```python
from build123d import *

# Parameters (mm, degrees)
SKETCH1_W                    = 68
SKETCH1_H                    = 40
BOSS_EXTRUDE1_DEPTH          = 3
SKETCH3_W                    = 50
SKETCH3_H                    = 42
BOSS_EXTRUDE2_DEPTH          = 3
CUT_EXTRUDE1_REACH           = 71.145
SKETCH4_R                    = 11.1
CSK_FOR_M3_SFHCS1_AT_2_COUNT = 2
CSK_FOR_M3_SFHCS1_AT_2_PITCH = 31
CSK_FOR_M3_SFHCS1_AT_3_COUNT = 2
CSK_FOR_M3_SFHCS1_AT_3_PITCH = 31
CSK_FOR_M3_SFHCS1_AT_4_COUNT = 2
CSK_FOR_M3_SFHCS1_AT_4_PITCH = 43.840620434
BOSS_EXTRUDE3_DEPTH          = 50
SKETCH9_W                    = 42.2
SKETCH9_H                    = 42
CUT_EXTRUDE2_DEPTH           = 37
FILLET1_R                    = 3
CSK_FOR_M3_SFHCS2_AT_2_COUNT = 2
CSK_FOR_M3_SFHCS2_AT_2_PITCH = 61.351446601
CSK_FOR_M3_SFHCS2_AT_3_COUNT = 2
CSK_FOR_M3_SFHCS2_AT_3_PITCH = 20
CSK_FOR_M3_SFHCS2_AT_4_COUNT = 2
CSK_FOR_M3_SFHCS2_AT_4_PITCH = 58


with BuildPart() as part:
    # Sketch1 → Boss-Extrude1 (new body)
    with BuildSketch(Plane.XY):
        with Locations((0, -20)):
            Rectangle(SKETCH1_W, SKETCH1_H)
    extrude(amount=BOSS_EXTRUDE1_DEPTH)

    # Sketch3 → Boss-Extrude2 (add)
    with BuildSketch(Plane(origin=(0, 0, 0), x_dir=(1, 0, 0), z_dir=(0, 1, 0))):
        with Locations((0, -24)):
            Rectangle(SKETCH3_W, SKETCH3_H)
    extrude(amount=-BOSS_EXTRUDE2_DEPTH)

    # Sketch4 → Cut-Extrude1 (cut, up to next)
    with BuildSketch(Plane(origin=(0, 0, 0), x_dir=(1, 0, 0), z_dir=(0, 1, 0)), mode=Mode.PRIVATE) as cut_extrude1_sk1:
        with Locations(Location((0, -24, 0), (0, 0, 180))):
            Circle(SKETCH4_R)
    cut_extrude1_tool1 = extrude(cut_extrude1_sk1.sketch, amount=-CUT_EXTRUDE1_REACH, mode=Mode.PRIVATE) & part.part
    add(cut_extrude1_tool1.solids().sort_by_distance((0, 0, 24))[0], mode=Mode.SUBTRACT)

    # Sketch6 → CSK for M3 SFHCS1 (revolve, cut)
    with BuildSketch(Plane(origin=(-15.5, 0, 8.5), x_dir=(0, 0, 1), z_dir=(1, 0, 0))):
        Polygon((0, 0), (0, 3), (1.7, 3), (1.7, 1.66), (3.36, 0), align=None)
    csk_for_m3_sfhcs1 = revolve(axis=Axis((-15.5, 6.35, 8.5), (0, -1, 0)), mode=Mode.SUBTRACT)

    # CSK for M3 SFHCS1 at 2: CSK for M3 SFHCS1 ×2
    with Locations(*[(i * CSK_FOR_M3_SFHCS1_AT_2_PITCH, 0, 0) for i in range(1, CSK_FOR_M3_SFHCS1_AT_2_COUNT)]):
        add(csk_for_m3_sfhcs1, mode=Mode.SUBTRACT)

    # CSK for M3 SFHCS1 at 3: CSK for M3 SFHCS1 ×2
    with Locations(*[(0, 0, i * CSK_FOR_M3_SFHCS1_AT_3_PITCH) for i in range(1, CSK_FOR_M3_SFHCS1_AT_3_COUNT)]):
        add(csk_for_m3_sfhcs1, mode=Mode.SUBTRACT)

    # CSK for M3 SFHCS1 at 4: CSK for M3 SFHCS1 ×2
    with Locations(*[Vector(0.7071067811865476, 0, 0.7071067811865476) * (i * CSK_FOR_M3_SFHCS1_AT_4_PITCH) for i in range(1, CSK_FOR_M3_SFHCS1_AT_4_COUNT)]):
        add(csk_for_m3_sfhcs1, mode=Mode.SUBTRACT)

    # Sketch7 → Boss-Extrude3 (add)
    with BuildSketch(Plane.ZY.offset(25)):
        Polygon((45, -3), (3, -36.75), (3, -3), align=None)
    extrude(amount=-BOSS_EXTRUDE3_DEPTH)

    # Sketch9 → Cut-Extrude2 (cut)
    with BuildSketch(Plane.XZ.offset(40)):
        with Locations((0, 24)):
            Rectangle(SKETCH9_W, SKETCH9_H)
    extrude(amount=-CUT_EXTRUDE2_DEPTH, mode=Mode.SUBTRACT)

    # Fillet1
    fillet1_edges = [part.edges().sort_by_distance(p)[0] for p in [
        (-25, -1.5, 45),
        (25, -1.5, 45),
    ]]
    fillet(fillet1_edges, radius=FILLET1_R)

    # Sketch11 → CSK for M3 SFHCS2 (revolve, cut)
    with BuildSketch(Plane(origin=(-29, -30, 3), x_dir=(0, -1, 0), z_dir=(1, 0, 0))):
        Polygon((0, 0), (0, 3), (1.7, 3), (1.7, 1.66), (3.36, 0), align=None)
    csk_for_m3_sfhcs2 = revolve(axis=Axis((-29, -30, 9.35), (0, 0, -1)), mode=Mode.SUBTRACT)

    # CSK for M3 SFHCS2 at 2: CSK for M3 SFHCS2 ×2
    with Locations(*[Vector(0.9453729816262721, 0.32599068331940423, 0) * (i * CSK_FOR_M3_SFHCS2_AT_2_PITCH) for i in range(1, CSK_FOR_M3_SFHCS2_AT_2_COUNT)]):
        add(csk_for_m3_sfhcs2, mode=Mode.SUBTRACT)

    # CSK for M3 SFHCS2 at 3: CSK for M3 SFHCS2 ×2
    with Locations(*[(0, i * CSK_FOR_M3_SFHCS2_AT_3_PITCH, 0) for i in range(1, CSK_FOR_M3_SFHCS2_AT_3_COUNT)]):
        add(csk_for_m3_sfhcs2, mode=Mode.SUBTRACT)

    # CSK for M3 SFHCS2 at 4: CSK for M3 SFHCS2 ×2
    with Locations(*[(i * CSK_FOR_M3_SFHCS2_AT_4_PITCH, 0, 0) for i in range(1, CSK_FOR_M3_SFHCS2_AT_4_COUNT)]):
        add(csk_for_m3_sfhcs2, mode=Mode.SUBTRACT)


solid = part.part
```
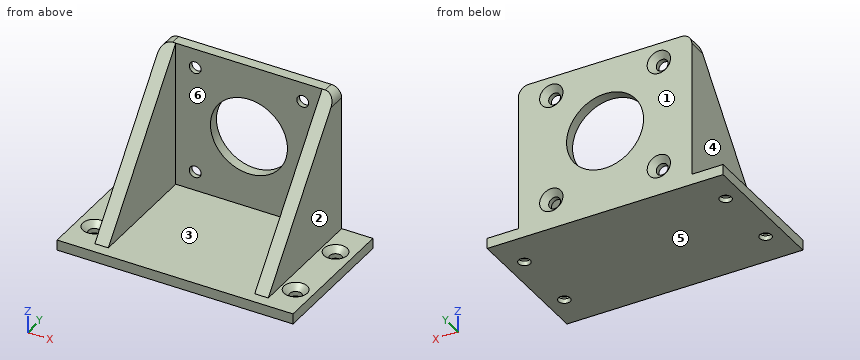
Work out the finished part from the listing and answer in its coordinate system (mm). Face numbers are marked on the shaded views. A direction names the side the tool comes from. Give positions to 0.01 mm unless a question says otherwise; leave off trailing zeros. Order: outer loops, then holes, each group sorted by start corner. A loop starts at its lowest first (then second) coordinate and runs counter-clockwise, first axis right, second up. Notation, with made-up numbers: (-7.75, -5.75) -> (36.25, -5.75) arc R24 cw to (36.25, 27.25) -> close; hole circle Ø9 at (80, -27). An arc over 180 degrees is marked (long way). Answer as CSV lines item,"result". Start each with the question number.
(1) Section C-C, the plane y = -34.5 is taken. Write down the section's boundary in (x, z).
(2) For a pull along X with two mould halves and no side action, classify the marked faces 1, 2 and 3 as released by +X, released by -X, zero draft, split by the parting line, or undercut.
(3) Each of these flat-tipped pins is pushed along its axis until it touches: pin 1 Ø12 at (y, z) = (-26.5, 13) entering from +X; pin 2 Ø5 at (x, y) = (-21.5, -22) entering from +Z; pin 3 Ø18.5 at (y, z) = (-26.5, 19) entering from -X. Where does it stop, or does it pass through?
(4) Section B-B, the plane x = -29 is taken. Write down the section's boundary in (y, z), plus the area to 3 significant figures.
(5) Section A-A, the plane y = -30 is taken. Write down the section's boundary in (x, z), plus the area to 3 significant figures.
(6) Consider line 1 along X through (y, z) = (-10, 0.7); line 2 along Z through (x, y) = (-15.5, -2.7); line 3 along Z through (x, y) = (0, -1). Determine where each line is inside the solid, lowest interval first.
(7) Section D-D, the plane x = -8.5 is taken. Write down the section's boundary in (y, z), plus the area to 3 significant figures.
(8) Which of the six approach directions +Z, -Z, +X, -X, +Y, -Y give full straight-line access (tool end or side, diameter ignored) to the marked faces 4, 5 and 6?
Entries:
1,outline,"(-34, 0) -> (34, 0) -> (34, 3) -> (25, 3) -> (25, 5.8) -> (21.1, 5.8) -> (21.1, 3) -> (-21.1, 3) -> (-21.1, 5.8) -> (-25, 5.8) -> (-25, 3) -> (-34, 3) -> close"
2,face 1,"zero draft"
2,face 2,"released by +X"
2,face 3,"undercut"
3,pin 1,"x = 25"
3,pin 2,"z = 24.47"
3,pin 3,"x = -25"
4,outline,"(-40, 0) -> (-31.7, 0) -> (-31.7, 1.34) -> (-33.36, 3) -> (-40, 3) -> close; (-28.3, 0) -> (-11.7, 0) -> (-11.7, 1.34) -> (-13.36, 3) -> (-26.64, 3) -> (-28.3, 1.34) -> close; (-8.3, 0) -> (0, 0) -> (0, 3) -> (-6.64, 3) -> (-8.3, 1.34) -> close"
4,area,"94.1 mm²"
5,outline,"(-34, 0) -> (-30.7, 0) -> (-30.7, 1.34) -> (-32.36, 3) -> (-34, 3) -> close; (-27.3, 0) -> (27.3, 0) -> (27.3, 1.34) -> (25.64, 3) -> (25, 3) -> (25, 11.4) -> (21.1, 11.4) -> (21.1, 3) -> (-21.1, 3) -> (-21.1, 11.4) -> (-25, 11.4) -> (-25, 3) -> (-25.64, 3) -> (-27.3, 1.34) -> close; (30.7, 0) -> (34, 0) -> (34, 3) -> (32.36, 3) -> (30.7, 1.34) -> close"
5,area,"244 mm²"
6,line 1,"-34 to -30.7, -27.3 to 27.3, 30.7 to 34"
6,line 2,"0 to 6.8, 10.2 to 37.8, 41.2 to 45"
6,line 3,"0 to 12.9, 35.1 to 45"
7,outline,"(-40, 0) -> (0, 0) -> (0, 16.86) -> (-3, 16.86) -> (-3, 3) -> (-40, 3) -> close; (-3, 31.14) -> (0, 31.14) -> (0, 45) -> (-3, 45) -> close"
7,area,"203 mm²"
8,face 4,"+Z, -X, +Y, -Y"
8,face 5,"-Z, +X, -X, +Y, -Y"
8,face 6,"+Z, -Y"
